Could you check a few things on this model? Use its own coordinates, in mm. Face numbers are marked on the shaded views. A direction names the side the tool comes from. Give positions to 0.01 mm unless a question says otherwise; leave off trailing zeros. Loops run counter-clockwise (first coordinate to the right, second up) from the corner with the lowest first, then second, coordinate; pieces in that order, holes last. Notation, with made-up numbers: M -32.5,18.25 L 21.5,18.25 A13 ccw 21.5,34.25 Z; hole C 9,18.5 d11. An arc over 180 degrees is marked long. Use a Markdown table: item, result. Add a question column.
1) Suppose I cut it at C-C on y = 1.5. List the corners of the cut face in (x, z) for me, and give its area (3 significant figures).
2) Which directions (+Z, -Z, +X, -X, +Y, -Y) give clear straight access to the entire face, cutting with the end or side of a thin tool? Please do the marked faces 5, 6, 7 and 8.
3) Suppose I cut it at A-A on x = 3. List the corners of the cut face in (y, z) for me.
4) Suppose I cut it at B-B on z = 2.25. List the corners of the cut face in (x, y) for me.
5) Will these pins go through, and if not, where does the flat tip stop? pin 1 Ø3 at (x, z) = (3.5, -1.5) entering from +Y; pin 2 Ø4 at (x, z) = (1.5, -1.5) entering from +Y; pin 3 Ø1.5 at (x, y) = (-2, 2) entering from -Z; pin 4 Ø0.6 at (x, y) = (3.5, 1.5) entering from +Z.
6) Suppose I cut it at D-D on z = 1. List the corners of the cut face in (x, y) for me.
7) We'd pull the mould along Z, two halves only. Please class the marked faces 1, 2, 3 and 4: +Z half, -Z half, draft (parallel to the pull), parting line (faces both ways), or undercut.
8) If I drill on line 1 along Z through (x, y) = (0, 0.9); line 2 along X through (y, z) = (1.7, -2.25); line 3 along X through (y, z) = (2.8, 0), over which ranges is the centre line in solid material (lowest first)? Write a range as [from, to].
Autodesk Inventor part; units mm, degrees
ref_plane "YZ Plane" through (0, 0, 0) normal (1, 0, 0) x (0, 1, 0)
ref_plane "XZ Plane" through (0, 0, 0) normal (0, 1, 0) x (-1, 0, 0)
ref_plane "XY Plane" through (0, 0, 0) normal (0, 0, 1) x (1, 0, 0)
sketch "Sketch2" plane through (0, 0, 0) normal (0, 1, 0) x (-1, 0, 0)
  circle A0 centre (0, 0) radius 4.8
  line L0 (1.618, 1.1756) -> (3.8833, 2.8214)
  line L1 (0.618, 1.9021) -> (1.4833, 4.5651)
  line L2 (-0.618, 1.9021) -> (-1.4833, 4.5651)
  line L3 (-1.618, 1.1756) -> (-3.8833, 2.8214)
  line L4 (-2, 0) -> (-4.8, 0)
  line L5 (1.618, -1.1756) -> (3.8833, -2.8214)
  line L6 (0.618, -1.9021) -> (1.4833, -4.5651)
  line L7 (-0.618, -1.9021) -> (-1.4833, -4.5651)
  line L8 (-1.618, -1.1756) -> (-3.8833, -2.8214)
  arc A1 (2, 0) -> (1.618, 1.1756) centre (0, 0) ccw
  arc A2 (0.618, -1.9021) -> (1.618, -1.1756) centre (0, 0) ccw
  arc A3 (-1.618, -1.1756) -> (-0.618, -1.9021) centre (0, 0) ccw
  arc A4 (0.618, 1.9021) -> (-0.618, 1.9021) centre (0, 0) ccw
  arc A5 (-1.618, 1.1756) -> (-2, 0) centre (0, 0) ccw
  line L9 (2, 0) -> (4.8, 0)
  dimension "d22" = 9.6
extrude "Extrusion1" add sketch "Sketch2" along normal blind 2 contours A0 L5 A2 L6 L7 A3 L8 L4 A5 L3 L2 A4 L1 L0 A1 L9
sketch "Sketch3" plane through (0, 2, 0) normal (0, 1, 0) x (1, 0, 0)
  circle A0 centre (0, 0) radius 2
  circle A1 centre (0, 0) radius 1.5
  dimension "d39" = 3
  dimension "d44" = 4
extrude "Extrusion2" add sketch "Sketch3" along normal blind 1 contours A0 | A1
extrude "Extrusion3" cut sketch "Sketch3" along normal blind 1 and the other way blind 2 contours A1
properties part number "Encoder_helice"
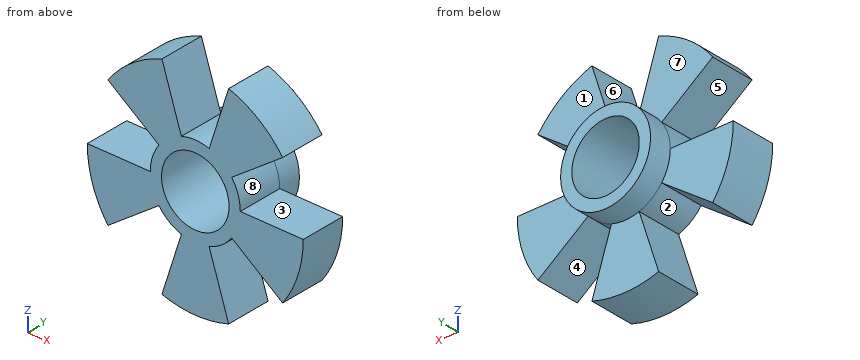
Answer block:
| question | item | result |
|---|---|---|
| 1 | outline | M -4.8,0 A4.8 ccw -3.88,-2.82 L -1.62,-1.18 A2 ccw -0.62,-1.9 L -1.48,-4.57 A4.8 ccw 1.48,-4.57 L 0.62,-1.9 A2 ccw 1.62,-1.18 L 3.88,-2.82 A4.8 ccw 4.8,0 L 2,0 A2 ccw 1.62,1.18 L 3.88,2.82 A4.8 ccw 1.48,4.57 L 0.62,1.9 A2 ccw -0.62,1.9 L -1.48,4.57 A4.8 ccw -3.88,2.82 L -1.62,1.18 A2 ccw -2,0 Z; hole C 0,0 d3 |
| 1 | area | 35.4 mm^2 |
| 2 | face 5 | -X, +Y, -Y |
| 2 | face 6 | +Z, +Y, -Y |
| 2 | face 7 | +Z, -X, +Y |
| 2 | face 8 | +X, +Y, -Y |
| 3 | outline | M 0,-2.18 L 2,-2.18 L 2,0 L 0,0 Z; M 0,2.18 L 2,2.18 L 2,3.75 L 0,3.75 Z |
| 4 | outline | M -3.1,0 L -0.73,0 L -0.73,2 L -3.1,2 Z; M 0.73,0 L 3.1,0 L 3.1,2 L 0.73,2 Z |
| 5 | pin 1 | stops at y = 2 |
| 5 | pin 2 | stops at y = 3 |
| 5 | pin 3 | stops at z = -4.63 |
| 5 | pin 4 | stops at z = 3.58 |
| 6 | outline | M -1.73,0 L -1.12,0 L -1.12,3 L -1.73,3 Z; M 1.12,0 L 1.73,0 L 1.73,3 L 1.12,3 Z |
| 7 | face 1 | draft |
| 7 | face 2 | undercut |
| 7 | face 3 | undercut |
| 7 | face 4 | -Z half |
| 8 | line 1 | z = [-4.8, -1.5], [1.5, 2] |
| 8 | line 2 | x = [-4.24, -3.1], [-0.73, 0.73], [3.1, 4.24] |
| 8 | line 3 | x = [-2, -1.5], [1.5, 2] |
